from build123d import *

# Parameters (mm, degrees)
SKETCH2_W                = 75
SKETCH2_H                = 30
BOSS_EXTRUDE1_DEPTH      = 8
SKETCH3_R                = 2.55
CUT_EXTRUDE1_DEPTH       = 7
SKETCH4_R                = 0.6
CUT_EXTRUDE2_DEPTH       = 1
LPATTERN3_COUNT          = 8
LPATTERN3_PITCH          = 8
BOSS_EXTRUDE2_DEPTH      = 5
BOSS_EXTRUDE2_DEPTH_BACK = 5
SKETCH5_W                = 30
SKETCH5_H                = 26
SKETCH6_W                = 30
SKETCH6_H                = 8
BOSS_EXTRUDE3_DEPTH      = 25
SKETCH8_W                = 25
SKETCH8_H                = 30
BOSS_EXTRUDE4_DEPTH      = 5
SKETCH9_W                = 30
SKETCH9_H                = 30
BOSS_EXTRUDE5_DEPTH      = 5
SKETCH11_R               = 11.1
CUT_EXTRUDE3_DEPTH       = 4
SKETCH13_R               = 1.5
CUT_EXTRUDE4_DEPTH       = 85.72307832
SKETCH16_W               = 30
SKETCH16_H               = 8
BOSS_EXTRUDE6_DEPTH      = 25
CUT_EXTRUDE5_DEPTH       = 81.486023631
CUT_EXTRUDE5_DEPTH_BACK  = 13
SKETCH14_R               = 2.5
SKETCH15_R               = 5
CUT_EXTRUDE6_DEPTH       = 85.72307832
FILLET2_R                = 10
FILLET3_R                = 10
CUT_EXTRUDE7_REACH       = 88.313
SKETCH18_R               = 7
SKETCH19_R               = 1.5
CUT_EXTRUDE8_DEPTH       = 101.169855745
SKETCH21_R               = 3.5
CUT_EXTRUDE9_DEPTH       = 3
SKETCH22_W               = 5
SKETCH22_H               = 30
CUT_EXTRUDE10_DEPTH      = 83.643814046


with BuildPart() as part:
    # Sketch2 → Boss-Extrude1 (new body)
    with BuildSketch(Plane(origin=(0, 0, 0), x_dir=(1, 0, 0), z_dir=(0, 1, 0))):
        with Locations((-34.5, 0)):
            Rectangle(SKETCH2_W, SKETCH2_H)
    extrude(amount=BOSS_EXTRUDE1_DEPTH)

    # Sketch3 → Cut-Extrude1 (cut)
    with BuildSketch(Plane(origin=(0, 8, 0), x_dir=(1, 0, 0), z_dir=(0, 1, 0))):
        with Locations(Location((0, 0, 0), (0, 0, 270))):
            Circle(SKETCH3_R)
    cut_extrude1 = extrude(amount=-CUT_EXTRUDE1_DEPTH, mode=Mode.SUBTRACT)

    # Sketch4 → Cut-Extrude2 (cut)
    with BuildSketch(Plane(origin=(0, 1, 0), x_dir=(1, 0, 0), z_dir=(0, 1, 0))):
        with Locations(Location((0, 0, 0), (0, 0, 270))):
            Circle(SKETCH4_R)
    cut_extrude2 = extrude(amount=-CUT_EXTRUDE2_DEPTH, mode=Mode.SUBTRACT)

    # LPattern3: Cut-Extrude1, Cut-Extrude2 ×8
    with Locations(*[(-i * LPATTERN3_PITCH, 0, 0) for i in range(1, LPATTERN3_COUNT)]):
        add(cut_extrude1, mode=Mode.SUBTRACT)
        add(cut_extrude2, mode=Mode.SUBTRACT)


with BuildPart() as body_2:
    # Mirror2: mirrored copy
    add(part.part.mirror(Plane(origin=(0, -5, 0), x_dir=(0, 0, 1), z_dir=(0, -1, 0))))


with BuildPart() as part_1:
    add(part.part)

    add(body_2.part)  # Boss-Extrude2 merges body 2
    # Sketch5 → Boss-Extrude2 (add, two sides: drawn at the far end of the back side and taken through both)
    with BuildSketch(Plane.ZY.offset(72).offset(-BOSS_EXTRUDE2_DEPTH_BACK)):
        with Locations((0, -5)):
            Rectangle(SKETCH5_W, SKETCH5_H)
    extrude(amount=BOSS_EXTRUDE2_DEPTH + BOSS_EXTRUDE2_DEPTH_BACK)

    # Sketch6 → Boss-Extrude3 (add)
    with BuildSketch(Plane(origin=(3, 0, 0), x_dir=(0, 0, -1), z_dir=(1, 0, 0))):
        with Locations((0, -14)):
            Rectangle(SKETCH6_W, SKETCH6_H)
    extrude(amount=BOSS_EXTRUDE3_DEPTH)

    # Sketch8 → Boss-Extrude4 (add)
    with BuildSketch(Plane.XZ.offset(18)):
        with Locations((15.5, 0)):
            Rectangle(SKETCH8_W, SKETCH8_H)
    extrude(amount=BOSS_EXTRUDE4_DEPTH)

    # Sketch9 → Boss-Extrude5 (add)
    with BuildSketch(Plane.XZ.offset(23)):
        with Locations((13, 0)):
            Rectangle(SKETCH9_W, SKETCH9_H)
    extrude(amount=BOSS_EXTRUDE5_DEPTH)

    # Sketch11 → Cut-Extrude3 (cut)
    with BuildSketch(Plane.XZ.offset(28)):
        with Locations(Location((11.5, 0, 0), (0, 0, 270))):
            Circle(SKETCH11_R)
    extrude(amount=-CUT_EXTRUDE3_DEPTH, mode=Mode.SUBTRACT)

    # Sketch13 → Cut-Extrude4 (cut, through all)
    with BuildSketch(Plane.XZ.offset(24)):
        with Locations(Location((11.5, 8.75, 0), (0, 0, 270))):
            Circle(SKETCH13_R)
        with Locations(Location((11.5, -8.75, 0), (0, 0, 270))):
            Circle(SKETCH13_R)
    extrude(amount=-CUT_EXTRUDE4_DEPTH, mode=Mode.SUBTRACT)

    # Sketch16 → Boss-Extrude6 (add)
    with BuildSketch(Plane(origin=(3, 0, 0), x_dir=(0, 0, -1), z_dir=(1, 0, 0))):
        with Locations((0, 4)):
            Rectangle(SKETCH16_W, SKETCH16_H)
    extrude(amount=BOSS_EXTRUDE6_DEPTH)

    # Sketch14 → Cut-Extrude5 (cut, two sides: drawn at the far end of the back side and taken through both)
    with BuildSketch(Plane(origin=(0, -10, 0), x_dir=(1, 0, 0), z_dir=(0, 1, 0)).offset(-CUT_EXTRUDE5_DEPTH_BACK)):
        with Locations(Location((11.5, 8.75, 0), (0, 0, 90))):
            Circle(SKETCH14_R)
        with Locations(Location((11.5, -8.75, 0), (0, 0, 90))):
            Circle(SKETCH14_R)
    extrude(amount=CUT_EXTRUDE5_DEPTH + CUT_EXTRUDE5_DEPTH_BACK, mode=Mode.SUBTRACT)

    # Sketch15 → Cut-Extrude6 (cut, through all)
    with BuildSketch(Plane.XZ.offset(24)):
        with Locations(Location((11.5, 0, 0), (0, 0, 270))):
            Circle(SKETCH15_R)
    extrude(amount=-CUT_EXTRUDE6_DEPTH, mode=Mode.SUBTRACT)

    # Fillet2
    fillet2_edges = [part_1.edges().sort_by_distance(p)[0] for p in [
        (28, -19, 15),
        (28, -19, -15),
    ]]
    fillet(fillet2_edges, radius=FILLET2_R)

    # Fillet3
    fillet3_edges = [part_1.edges().sort_by_distance(p)[0] for p in [
        (28, 4, 15),
        (28, 4, -15),
    ]]
    fillet(fillet3_edges, radius=FILLET3_R)

    # Sketch18 → Cut-Extrude7 (cut, up to next)
    with BuildSketch(Plane(origin=(0, 8, 0), x_dir=(1, 0, 0), z_dir=(0, 1, 0)), mode=Mode.PRIVATE) as cut_extrude7_sk1:
        with Locations((11.5, 0)):
            Circle(SKETCH18_R)
    cut_extrude7_tool1 = extrude(cut_extrude7_sk1.sketch, amount=-CUT_EXTRUDE7_REACH, mode=Mode.PRIVATE) & part_1.part
    add(cut_extrude7_tool1.solids().sort_by_distance((11.5, 8, 0))[0], mode=Mode.SUBTRACT)

    # Sketch19 → Cut-Extrude8 (cut, through all)
    with BuildSketch(Plane(origin=(-67, 0, 0), x_dir=(0, 0, -1), z_dir=(1, 0, 0))):
        with Locations((0, -5)):
            Circle(SKETCH19_R)
    extrude(amount=-CUT_EXTRUDE8_DEPTH, mode=Mode.SUBTRACT)

    # Sketch21 → Cut-Extrude9 (cut)
    with BuildSketch(Plane(origin=(-67, 0, 0), x_dir=(0, 0, -1), z_dir=(1, 0, 0))):
        with Locations((0, -5)):
            Circle(SKETCH21_R)
    extrude(amount=-CUT_EXTRUDE9_DEPTH, mode=Mode.SUBTRACT)

    # Sketch22 → Cut-Extrude10 (cut, through all)
    with BuildSketch(Plane.XZ.offset(18)):
        with Locations((0.5, 0)):
            Rectangle(SKETCH22_W, SKETCH22_H)
    extrude(amount=CUT_EXTRUDE10_DEPTH, mode=Mode.SUBTRACT)


solid = part_1.part
Work out the finished part from the listing and answer in its coordinate system (mm). A direction names the side the tool comes from. Coordinates: 2 decimals unless noted, no trailing zeros. Write each loop counter-clockwise with the first axis right and the second up, starting at its lowest first coordinate (ties: lowest second). Pieces come first, ordered by that corner, then holes. Notation, with made-up numbers: (49, 13) - (77, 13) arc R23 cw to (77, 49) - close; hole circle Ø1 at (3.5, 35). An arc over 180 degrees is marked (long way). One line per question, with ' | ' between items.
1) Find section D-D, the plane z = 13. Determine the outline of the cut face in (x, y).
Checks:
outline: (-77, -18) - (3, -18) - (3, -28) - (24, -28) - (24, -10) - (-67, -10) - (-67, 0) - (24, 0) - (24, 8) - (-77, 8) - close
2) Find section C-C, the plane y = -21.5. Determine the outline of the cut face in (x, z).
Checks:
outline: (3, -15) - (18, -15) arc R10 ccw to (28, -5) - (28, 5) arc R10 ccw to (18, 15) - (3, 15) - close; hole circle Ø10 at (11.5, 0); hole circle Ø5 at (11.5, -8.75); hole circle Ø5 at (11.5, 8.75)
3) For faces 4 (the face through (3, -22, 0)), 5 (the face through (-68.479, -8.417, 0.759)), 6 (the face through (-45.47, 4.55, -0.33)), determine the directions among +Z, -Z, +X, -X, +Y, -Y from which every point of the face is accessible in a straight line to the end or side of a thin tool.
Checks:
face 4: +Z, -Z, -X, -Y | face 5: +X | face 6: +Y
4) Flat-ended cylindrical pins translate along their axes: P1, Ø4, axis at x = -8, z = 0, coming from the +Y side; P2, Ø15.5, axis at x = 10, z = -2.5, coming from the -Y side; P3, Ø5.5, axis at x = -16.5, z = 0, coming from the +Y side; P4, Ø8, axis at x = -51, z = 2, coming from the -Y side. Find the tip coordinate at first contact, or state that the pin passes through.
Checks:
P1: y = 1 | P2: y = -24 | P3: y = 8 | P4: y = -18
5) Find section B-B, the plane x = -64.5. Determine the outline of the cut face in (y, z).
Checks:
outline: (-18, -15) - (-10, -15) - (-10, 15) - (-18, 15) - close; (0, -15) - (8, -15) - (8, 15) - (0, 15) - close
6) Find section A-A, the plane y = -5. Determine the outline of the cut face in (x, z), and give its area (3 significant figures).
Checks:
outline: (-77, -15) - (-67, -15) - (-67, -3.5) - (-70, -3.5) - (-70, -1.5) - (-77, -1.5) - close; (-77, 1.5) - (-70, 1.5) - (-70, 3.5) - (-67, 3.5) - (-67, 15) - (-77, 15) - close | area: 258 mm2
7) Consider probe 1 along Y at (x, z) = (-18.5, -5); probe 2 along Y at (x, z) = (21, 12); probe 3 along Z at (x, y) = (11.5, -25.5). Determine where each line is inside the solid, lowest interval first. Write a range as [from, to].
Checks:
probe 1: [-18, -10], [0, 8] | probe 2: [-28, -10], [0, 8] | probe 3: [-15, -11.1], [11.1, 15]
8) The mould has two halves that part along Y. Classify faces 1 (the face through (-70, -7, 0)), 2 (the face through (-7, -11, 0)), 3 (the face through (22.594, -26.028, -0.38)): +Y half, -Y half, draft (parallel to the pull), parting line (faces both ways), or undercut.
Checks:
face 1: undercut | face 2: -Y half | face 3: draft
